```python
from build123d import *

# Parameters (mm, degrees)
F1_DEPTH = 44.45
F3_DEPTH = 44.451
F5_DEPTH = 38.101
F6_R     = 5.08
F7_R     = 5.08
F8_R     = 2.54


with BuildPart() as f1:
    # F0 (on Front) → F1 (new body)
    with BuildSketch(Plane.XZ):
        Polygon((19.05, -31.75), (19.05, 31.75), (-19.05, 31.75), (-19.05, 0), (-19.05, -31.75), align=None)
        with BuildLine():
            ThreePointArc((-6.35, 0), (-9.525, -3.175), (-12.7, 0))
            ThreePointArc((-12.7, 0), (-9.525, 3.175), (-6.35, 0))
        make_face(mode=Mode.SUBTRACT)
    extrude(amount=F1_DEPTH)

    # F2 (on face) → F3 (cut, through all)
    with BuildSketch(Plane(origin=(0, 0, 0), x_dir=(-1, 0, 0), z_dir=(0, 1, 0))):
        with BuildLine():
            ThreePointArc((-12.7, -15.875), (-8.980256, -24.855256), (0, -28.575))
            Line((0, -28.575), (0, -15.875))
            Line((0, -15.875), (-12.7, -15.875))
        make_face()
        with BuildLine():
            Line((0, -15.875), (0, -28.575))
            ThreePointArc((0, -28.575), (8.980256, -24.855256), (12.7, -15.875))
            Line((12.7, -15.875), (0, -15.875))
        make_face()
        with BuildLine():
            ThreePointArc((11.43, 14.6812), (-8.082231, 22.763431), (0, 3.2512))
            ThreePointArc((0, 3.2512), (8.082231, 6.598969), (11.43, 14.6812))
        make_face()
        with BuildLine():
            Line((-12.7, -15.875), (0, -15.875))
            Line((0, -15.875), (0, -3.175))
            ThreePointArc((0, -3.175), (-8.980256, -6.894744), (-12.7, -15.875))
        make_face()
        with BuildLine():
            Line((0, -3.175), (0, -15.875))
            Line((0, -15.875), (12.7, -15.875))
            ThreePointArc((12.7, -15.875), (8.980256, -6.894744), (0, -3.175))
        make_face()
    extrude(amount=-F3_DEPTH, mode=Mode.SUBTRACT)

    # F4 (on face) → F5 (cut, through all)
    with BuildSketch(Plane.YZ.offset(19.05)):
        Polygon((-22.86, 3.2512), (-9.652, 3.2512), (-13.462, 10.3632), (-26.67, 10.3632), align=None)
    extrude(amount=-F5_DEPTH, mode=Mode.SUBTRACT)

    # F6
    f6_edges = [f1.edges().sort_by_distance(p)[0] for p in [
        (-19.05, -22.225, 31.75),
        (19.05, -22.225, 31.75),
    ]]
    fillet(f6_edges, radius=F6_R)

    # F7
    f7_edges = [f1.edges().sort_by_distance(p)[0] for p in [
        (19.05, -22.225, -31.75),
        (-19.05, -22.225, -31.75),
    ]]
    fillet(f7_edges, radius=F7_R)

    # F8
    f8_edges = [f1.edges().sort_by_distance(p)[0] for p in [
        (0, 0, 31.75),
    ]]
    fillet(f8_edges, radius=F8_R)


solid = f1.part
```
Input: part model. Units: mm. Frame: model coordinates. A direction names the side the tool comes from. Give positions to 0.01 mm unless a question says otherwise; leave off trailing zeros. Write each loop counter-clockwise with the first axis right and the second up, starting at its lowest first coordinate (ties: lowest second). Pieces come first, ordered by that corner, then holes. Notation, with made-up numbers: (-28.5, 29.25) - (22.5, 29.25) arc R16 cw to (22.5, 59.25) - close; hole circle Ø1 at (31.5, 17.5). An arc over 180 degrees is marked (long way). Write item = value, one per line. Start each with the question number.
1) Material intervals for L1, parallel to X at y = -26, z = 22; L2, parallel to Z at x = -9, y = -2; L3, parallel to X at y = -9, z = -0.5, sorted ascending. Write a range as [from, to].
2) Cut plane A-A (y = -16.5). Return loops of the section in (x, z) (3 decimals), and give its area (3 significant figures).
3) Cut plane D-D (z = 8). Return loops of the section in (x, y).
4) Draft query along Z for faces 1 (the face through (-13.625, -24.792, 6.857)), 2 (the face through (0, -44.45, 0)), 3 (the face through (-17.522, -23.788, 30.301)). Return one class per face: pulls with the +Z half, pulls with the -Z half, needs draft (parallel to the pull), parting line crosses it, or undercut.
5) Pin query (flat end, axial travel): pin 1 (5.5 mm diameter, centred on x = -9.525, z = 0, fed in from +Y). Return the tip coordinate at first contact, or that it passes through.
6) Reachability of faces 4 (the face through (19.05, -23, 0)), 5 (the face through (0, -16, 3.251)) from +Z, -Z, +X, -X, +Y, -Y: full face, straight path, thin tool, end or side. Return the list, or none.
7) Cut plane C-C (y = -36). Return loops of the section in (x, z) (3 decimals).
8) Cut plane B-B (z = 0). Return loops of the section in (x, y), and give its area (3 significant figures).
Answers follow:
q1.L1 = [-19.05, -8.78], [8.78, 19.05]
q1.L2 = [-31.69, -24.84], [-6.91, -3.13], [3.13, 7.64], [21.73, 31.69]
q1.L3 = [-19.05, -12.66], [-6.39, 19.05]
q2.outline = (-19.05, -26.67) arc R5.08 ccw to (-13.97, -31.75) - (13.97, -31.75) arc R5.08 ccw to (19.05, -26.67) - (19.05, 3.251) - (-19.05, 3.251) - close; (-19.05, 10.363) - (-10.583, 10.363) arc R11.43 cw to (-11.43, 14.681) arc R11.43 cw (long way) to (10.583, 10.363) - (19.05, 10.363) - (19.05, 26.67) arc R5.08 ccw to (13.97, 31.75) - (-13.97, 31.75) arc R5.08 ccw to (-19.05, 26.67) - close; hole circle Ø25.4 at (0, -15.875); hole circle Ø6.35 at (-9.525, 0)
q2.area = 1,290 mm^2
q3.outline = (-19.05, -44.45) - (-9.27, -44.45) - (-9.27, -25.4) - (-19.05, -25.4) - close; (-19.05, -12.2) - (-9.27, -12.2) - (-9.27, 0) - (-16.51, 0) arc R2.54 ccw to (-19.05, -2.54) - close; (9.27, -44.45) - (19.05, -44.45) - (19.05, -25.4) - (9.27, -25.4) - close; (9.27, -12.2) - (19.05, -12.2) - (19.05, -2.54) arc R2.54 ccw to (16.51, 0) - (9.27, 0) - close
q4.face_1 = undercut
q4.face_2 = needs draft
q4.face_3 = pulls with the +Z half
q5.pin_1 = through
q6.face_4 = +Z, -Z, +X, +Y, -Y
q6.face_5 = +X, -X
q7.outline = (-19.05, -26.67) arc R5.08 ccw to (-13.97, -31.75) - (13.97, -31.75) arc R5.08 ccw to (19.05, -26.67) - (19.05, 26.67) arc R5.08 ccw to (13.97, 31.75) - (-13.97, 31.75) arc R5.08 ccw to (-19.05, 26.67) - close; hole circle Ø25.4 at (0, -15.875); hole circle Ø6.35 at (-9.525, 0); hole (-11.43, 14.681) arc R11.43 ccw to (0, 3.251) arc R11.43 ccw (long way) to start
q8.outline = (-19.05, -44.45) - (-12.7, -44.45) - (-12.7, 0) - (-16.51, 0) arc R2.54 ccw to (-19.05, -2.54) - close; (-6.35, -44.45) - (19.05, -44.45) - (19.05, -2.54) arc R2.54 ccw to (16.51, 0) - (-6.35, 0) - close
q8.area = 1,410 mm^2
